Could you check a few things on this drawing? It's one solid part, dimensions in mm from its lowest x, y, z. A direction names the side the tool comes from. Coordinates: 2 decimals unless noted, no trailing zeros. Order: outer loops, then holes, each group sorted by start corner. A loop starts at its lowest first (then second) coordinate and runs counter-clockwise, first axis right, second up.
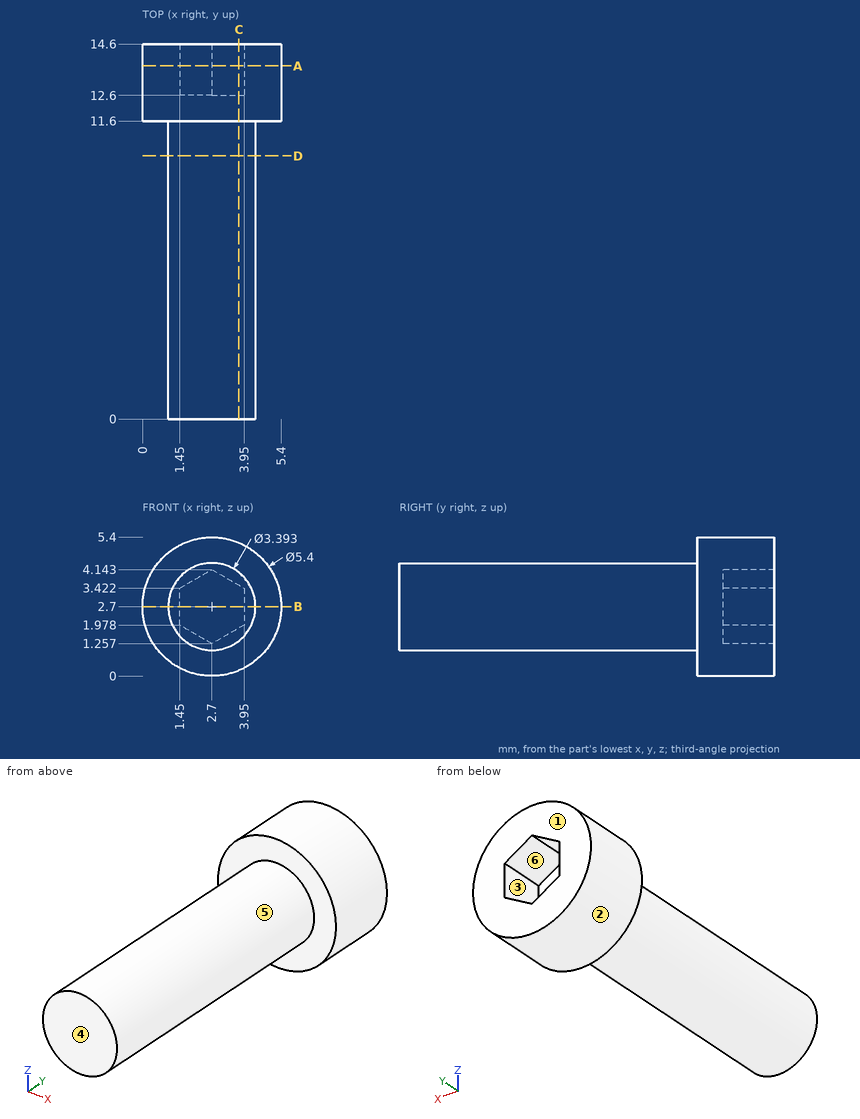
1. Imagine slicing it at C-C on x = 3.75. Please give me the cut outline in (y, z).
Completed:
outline: (0, 1.37) - (11.6, 1.37) - (11.6, 0.21) - (14.6, 0.21) - (14.6, 1.86) - (12.6, 1.86) - (12.6, 3.54) - (14.6, 3.54) - (14.6, 5.19) - (11.6, 5.19) - (11.6, 4.03) - (0, 4.03) - close
2. Thinking about a two-plate mould opening in X: for the marked faces 1, 2 and 3, which applies, pulls with the +X half, pulls with the -X half, needs draft (parallel to the pull), parting line crosses it, or undercut?
Completed:
face 1: needs draft
face 2: parting line crosses it
face 3: undercut
3. On a 3-axis mill with a long thin cutter (end or side, diameter ignored), from which of +Z, -Z, +X, -X, +Y, -Y can I reach the whole of each face in a straight line? I mean the marked faces 4, 5 and 6. Say none if no direction works.
Completed:
face 4: +Z, -Z, +X, -X, -Y
face 5: -Y
face 6: +Y
4. Imagine slicing it at A-A on y = 13.75. Please give me the cut outline in (x, z), then the cut area to 3 significant figures.
Completed:
outline: circle Ø5.4 at (2.7, 2.7); hole (1.45, 1.98) - (2.7, 1.26) - (3.95, 1.98) - (3.95, 3.42) - (2.7, 4.14) - (1.45, 3.42) - close
area: 17.5 mm2
5. Please list where these lines run through material, in increasing order: probe 1 along Y at (x, z) = (0.4, 2.85); probe 2 along Y at (x, z) = (3.4, 2.9); probe 3 along Z at (x, y) = (2.15, 11.5) (1 decimal).
Completed:
probe 1: y = 11.6 to 14.6
probe 2: y = 0 to 12.6
probe 3: z = 1.1 to 4.3
6. Imagine slicing it at B-B on z = 2.7. Please give me the cut outline in (x, y).
Completed:
outline: (0, 11.6) - (1, 11.6) - (1, 0) - (4.4, 0) - (4.4, 11.6) - (5.4, 11.6) - (5.4, 14.6) - (3.95, 14.6) - (3.95, 12.6) - (1.45, 12.6) - (1.45, 14.6) - (0, 14.6) - close
7. I'm going to push flat-ended pins straight in: pin 1 (0.8 mm diameter, centred on x = 2.5, z = 2, fed in from +Y); pin 2 (1.5 mm diameter, centred on x = 2.5, y = 5, fed in from -Z); pin 3 (1.5 mm diameter, centred on y = 13, z = 4.5, fed in from +X). Where does each tip first touch, or does it pass through?
Completed:
pin 1: stops at y = 12.6
pin 2: stops at z = 1
pin 3: stops at x = 5.19
8. Imagine slicing it at D-D on y = 10.25. Please give me the cut outline in (x, z).
Completed:
outline: circle Ø3.39 at (2.7, 2.7)
